Can you work these out from the model? Positions are in its coordinate system, mm. Coordinates: 2 decimals unless noted, no trailing zeros. Order: outer loops, then holes, each group sorted by start corner. A loop starts at its lowest first (then second) coordinate and runs counter-clockwise, first axis right, second up. Notation, with made-up numbers: (11.5, 34) - (65.5, 34) arc R19 ccw to (65.5, 68) - close; hole circle Ø11 at (27, 82). An arc over 180 degrees is marked (long way). Return JSON: item names as keys, results as strings. Group by question number.
1) If I drill on line 1 along Z through (x, y) = (-27, -0.5); line 2 along Y through (x, z) = (-27, 0.25); line 3 along Z through (x, y) = (-52.5, -2.5), over which ranges is the centre line in solid material (lowest first)?
2) Imagine slicing it at B-B (x = -66). Write out the boundary of the cut face in (y, z).
3) Imagine slicing it at A-A (x = -42). Write out the boundary of the cut face in (y, z).
4) For pin 1 Ø2 at (x, y) = (-55, -3.5) entering from -Z; pin 2 Ø3 at (x, y) = (-76.5, 0.5) entering from -Z; pin 3 Ø6 at (x, y) = (-11, 1.5) entering from +Z; pin 4 Ø1 at (x, y) = (-36, -1.5) entering from -Z, each with a flat end and sliding along its axis, tell me the tip position at first contact or that it passes through.
```python
from build123d import *


with BuildPart() as part:
    # Esquisse1 → Révolution1 (revolve)
    with BuildSketch(Plane.XY):
        with BuildLine():
            Line((0, 0), (0, 3.5))
            ThreePointArc((0, 3.5), (-0.439339828, 4.560660172), (-1.5, 5))
            Line((-1.5, 5), (-55, 5))
            Line((-55, 5), (-55, 4.99))
            Line((-55, 4.99), (-84, 4.99))
            Line((-84, 4.99), (-85, 3.99))
            Line((-85, 3.99), (-85, 0))
            Line((-85, 0), (0, 0))
        make_face()
    revolve(axis=Axis((-85, 0, 0), (1, 0, 0)))


solid = part.part
```
Calculated:
{
 "1": {"line 1": "-4.97 to 4.97", "line 2": "-4.99 to 4.99", "line 3": "-4.33 to 4.33"},
 "2": {"outline": "circle Ø9.98 at (0, 0)"},
 "3": {"outline": "circle Ø10 at (0, 0)"},
 "4": {"pin 1": "z = -4.33", "pin 2": "z = -4.99", "pin 3": "z = 5", "pin 4": "z = -4.9"}
}
